Design review of the part built by this model. Coordinates are the model's own, in mm. A direction names the side the tool comes from. Round coordinates to 2 decimals unless told otherwise and drop trailing zeros. Loops run counter-clockwise (first coordinate to the right, second up) from the corner with the lowest first, then second, coordinate; pieces in that order, holes last. Notation, with made-up numbers: (38.25, -11) -> (55.25, -11) arc R33 ccw to (55.25, 17) -> close; hole circle Ø11 at (1, 39.25). An arc over 180 degrees is marked (long way). Answer as CSV lines item,"result". Start each with the question number.
```python
from build123d import *

# Parameters (mm, degrees)
SKETCH1_W           = 500
SKETCH1_H           = 900
BOSS_EXTRUDE1_DEPTH = 20
CHAMFER1_SIZE       = 50
SKETCH2_R           = 10
CUT_EXTRUDE1_DEPTH  = 516.169874896
SKETCH3_R           = 100
BOSS_EXTRUDE2_DEPTH = 125
SKETCH4_R           = 10
CUT_EXTRUDE2_DEPTH  = 530.74050251


with BuildPart() as part:
    # Sketch1 → Boss-Extrude1 (new body)
    with BuildSketch(Plane(origin=(0, 0, 0), x_dir=(1, 0, 0), z_dir=(0, 1, 0))):
        Rectangle(SKETCH1_W, SKETCH1_H)
    extrude(amount=BOSS_EXTRUDE1_DEPTH)

    # Chamfer1
    chamfer1_edges = [part.edges().sort_by_distance(p)[0] for p in [
        (-250, 10, -450),
        (250, 10, -450),
    ]]
    chamfer(chamfer1_edges, length=CHAMFER1_SIZE)

    # Sketch2 → Cut-Extrude1 (cut, through all)
    with BuildSketch(Plane(origin=(0, 20, 0), x_dir=(1, 0, 0), z_dir=(0, 1, 0))):
        with Locations(Location((200, 230, 0), (0, 0, 270))):
            Circle(SKETCH2_R)
        with Locations(Location((-200, 230, 0), (0, 0, 270))):
            Circle(SKETCH2_R)
        with Locations(Location((200, -270, 0), (0, 0, 270))):
            Circle(SKETCH2_R)
        with Locations(Location((-200, -270, 0), (0, 0, 270))):
            Circle(SKETCH2_R)
    extrude(amount=-CUT_EXTRUDE1_DEPTH, mode=Mode.SUBTRACT)

    # Sketch3 → Boss-Extrude2 (add)
    with BuildSketch(Plane(origin=(0, 20, 0), x_dir=(1, 0, 0), z_dir=(0, 1, 0))):
        with Locations(Location((0, 0, 0), (0, 0, 270))):
            Circle(SKETCH3_R)
    extrude(amount=BOSS_EXTRUDE2_DEPTH)

    # Sketch4 → Cut-Extrude2 (cut, through all)
    with BuildSketch(Plane(origin=(0, 20, 0), x_dir=(1, 0, 0), z_dir=(0, 1, 0))):
        with Locations(Location((0, -400, 0), (0, 0, 270))):
            Circle(SKETCH4_R)
    extrude(amount=-CUT_EXTRUDE2_DEPTH, mode=Mode.SUBTRACT)


solid = part.part
```
Q1. Mouldability with a two-part tool opening along Z and no side actions: class faces 3 (the cylindrical face through (203, 10.14, 279.54)), 4 (the flat face through (250, 10, 31)), 5 (the flat face through (-3, 10, 450)) as pulls with the +Z half, pulls with the -Z half, needs draft (parallel to the pull), parting line crosses it, or undercut.
Q2. Add section C-C, the plane x = -89.5. Give the boundary of the cut face in (y, z).
Q3. Add section B-B, the plane z = -10.5. Give the boundary of the cut face in (x, y), and give its area (3 significant figures).
Q4. Add section A-A, the plane x = 0. Give the boundary of the cut face in (y, z), and give its area (3 significant figures).
Q5. To check wall thickness, follow probe 1 along X at (y, z) = (8.5, -230); probe 2 along Y at (x, z) = (-155, 332); probe 3 along X at (y, z) = (35, -2). State the ranges of each line that lie inside material, in increasing order. Write a range as from..to.
Q6. Add section D-D, the plane y = 110.5. Give the boundary of the cut face in (x, z), and give its area (3 significant figures).
Q7. Machinability: for faces 1 (the cylindrical face through (30.04, 81.62, 95.38)), 2 (the flat face through (-3, 10, -450)), which of the approach directions +Z, -Z, +X, -X, +Y, -Y give a long, thin tool a straight path to every point of the face, cutting with its end or side? Answer none if there is none.
Q8. For pin 1 Ø4 at (x, z) = (-79, 40) entering from -Y; pin 2 Ø1 at (y, z) = (27, -19.5) entering from -X; pin 3 Ø12 at (x, z) = (66, 87.5) entering from +Y; pin 4 Ø10 at (y, z) = (57, 36) entering from -X, all flat-tipped, find the tip position at first contact; note any pin that passes through.
Worked answers:
1,face 3,"undercut"
1,face 4,"needs draft"
1,face 5,"pulls with the +Z half"
2,outline,"(0, -450) -> (20, -450) -> (20, -44.61) -> (145, -44.61) -> (145, 44.61) -> (20, 44.61) -> (20, 450) -> (0, 450) -> close"
3,outline,"(-250, 0) -> (250, 0) -> (250, 20) -> (99.45, 20) -> (99.45, 145) -> (-99.45, 145) -> (-99.45, 20) -> (-250, 20) -> close"
3,area,"34,900 mm^2"
4,outline,"(0, -450) -> (20, -450) -> (20, -100) -> (145, -100) -> (145, 100) -> (20, 100) -> (20, 390) -> (0, 390) -> close; (0, 410) -> (20, 410) -> (20, 450) -> (0, 450) -> close"
4,area,"42,600 mm^2"
5,probe 1,"x = -250..-210, -190..190, 210..250"
5,probe 2,"y = 0..20"
5,probe 3,"x = -99.98..99.98"
6,outline,"circle Ø200 at (0, 0)"
6,area,"31,400 mm^2"
7,face 1,"+Y"
7,face 2,"-Z, +X, -X, +Y, -Y"
8,pin 1,"stops at y = 0"
8,pin 2,"stops at x = -98.18"
8,pin 3,"stops at y = 20"
8,pin 4,"stops at x = -95.07"
